Source: CAD feature listing. Evaluate the final solid. Frame: model axes, mm. Face numbers are marked on the shaded views. Coordinates: 2 decimals unless noted, no trailing zeros. Write each loop counter-clockwise with the first axis right and the second up, starting at its lowest first coordinate (ties: lowest second). Pieces come first, ordered by that corner, then holes. Notation, with made-up numbers: M 32,-39 L 40,-39 A17 ccw 40,-33 Z; hole C -5.75,33 d9. An arc over 180 degrees is marked long. One line per item, written item: value. Start each with the question number.
Item 1: Cut plane A-A, the plane x = 6.5. Output: boundary loops of the cut face in (y, z).
Item 2: Cut plane B-B, the plane z = -63.5. Output: boundary loops of the cut face in (x, y).
Item 3: Ray query, L1, parallel to Y at x = 34, z = 26.5; L2, parallel to Y at x = -28, z = -60. Return the intervals inside material, ascending. Write a range as from..to.
Item 4: Cut plane C-C, the plane x = -9. Output: boundary loops of the cut face in (y, z), then the cut area to 3 significant figures.
Item 5: Pin query (flat end, axial travel): P1, Ø1.9, axis at y = -97, z = -63.5, coming from the -X side; P2, Ø5, axis at y = 107, z = -40, coming from the -X side; P3, Ø4.5, axis at x = 5, z = -64, coming from the -Y side. Return the tip coordinate at first contact, or that it passes through.
Item 6: Mould query, pull axis Y, two halves, no side actions, for the marked faces 1, 2 and 3. Classes: released by +Y, released by -Y, zero draft, split by the parting line, or undercut.
Item 7: Cut plane D-D, the plane z = 33. Output: boundary loops of the cut face in (x, y), then the cut area to 3 significant figures.
```python
from build123d import *

# Parameters (mm, degrees)
F0_W     = 85
F0_H     = 165
F1_DEPTH = 100
F2_W     = 30
F2_H     = 32
F3_DEPTH = 10
F4_W     = 85
F4_H     = 35
F5_DEPTH = 5.7
F6_R     = 7.5
F7_DEPTH = 2.6
F8_W     = 15
F8_H     = 20
F9_DEPTH = 6.2


with BuildPart() as f1:
    # F0 (on Front) → F1 (new body, symmetric)
    with BuildSketch(Plane.XZ):
        Rectangle(F0_W, F0_H)
    extrude(amount=F1_DEPTH, both=True)

    # F2 (on face) → F3 (join)
    with BuildSketch(Plane(origin=(0, 100, 0), x_dir=(-1, 0, 0), z_dir=(0, 1, 0))):
        with Locations((15.5, -43.5)):
            Rectangle(F2_W, F2_H)
    extrude(amount=F3_DEPTH)

    # F4 (on face) → F5 (cut)
    with BuildSketch(Plane.XZ.offset(100)):
        with Locations((0, -65)):
            Rectangle(F4_W, F4_H)
    extrude(amount=-F5_DEPTH, mode=Mode.SUBTRACT)

    # F6 (on face) → F7 (join)
    with BuildSketch(Plane.XZ.offset(94.3)):
        with Locations((6.5, -63.5)):
            Circle(F6_R)
        with Locations((26.5, -63.5)):
            Circle(F6_R)
    extrude(amount=F7_DEPTH)

    # F8 (on face) → F9 (join)
    with BuildSketch(Plane.XZ.offset(94.3)):
        with Locations((-20, -62.5)):
            Rectangle(F8_W, F8_H)
    extrude(amount=F9_DEPTH)


solid = f1.part
```
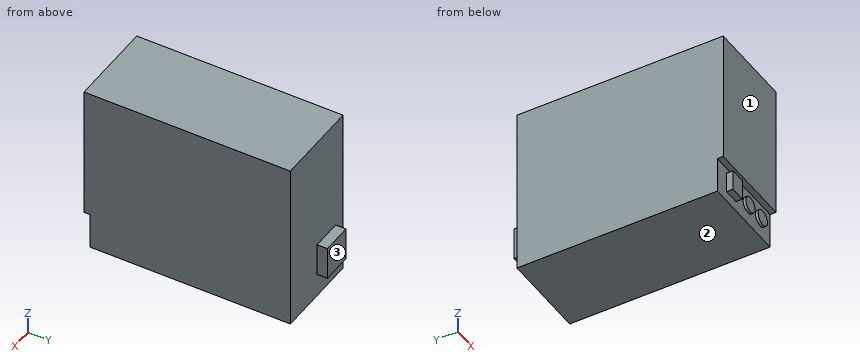
From the geometry:
1. outline: M -100,-47.5 L -94.3,-47.5 L -94.3,-56 L -96.9,-56 L -96.9,-71 L -94.3,-71 L -94.3,-82.5 L 100,-82.5 L 100,82.5 L -100,82.5 Z
2. outline: M -42.5,-94.3 L -27.5,-94.3 L -27.5,-100.5 L -12.5,-100.5 L -12.5,-94.3 L -1,-94.3 L -1,-96.9 L 14,-96.9 L 14,-94.3 L 19,-94.3 L 19,-96.9 L 34,-96.9 L 34,-94.3 L 42.5,-94.3 L 42.5,100 L -42.5,100 Z
3. L1: y = -100..100
3. L2: y = -94.3..100
4. outline: M -100,-47.5 L -94.3,-47.5 L -94.3,-82.5 L 100,-82.5 L 100,-59.5 L 110,-59.5 L 110,-27.5 L 100,-27.5 L 100,82.5 L -100,82.5 Z
4. area: 33,100 mm²
5. P1: stops at x = -27.5
5. P2: stops at x = -30.5
5. P3: stops at y = -96.9
6. face 1: released by -Y
6. face 2: zero draft
6. face 3: released by +Y
7. outline: M -42.5,-100 L 42.5,-100 L 42.5,100 L -42.5,100 Z
7. area: 17,000 mm²
